Source: CAD feature listing. Evaluate the final solid. Frame: model axes, mm. A direction names the side the tool comes from. Coordinates: 2 decimals unless noted, no trailing zeros. Write each loop counter-clockwise with the first axis right and the second up, starting at its lowest first coordinate (ties: lowest second). Pieces come first, ordered by that corner, then holes. Notation, with made-up numbers: (4.25, 61) -> (58.25, 61) arc R16 cw to (58.25, 86) -> close; hole circle Ø4 at (38.5, 62.5). An arc over 180 degrees is marked (long way). Write item = value, one per line.
from build123d import *

# Parameters (mm, degrees)
SKETCH1_W           = 125
SKETCH1_H           = 125
SKETCH1_W_2         = 121
SKETCH1_H_2         = 121
BOSS_EXTRUDE1_DEPTH = 70
SKETCH2_W           = 125
SKETCH2_H           = 125
BOSS_EXTRUDE2_DEPTH = 2
SKETCH3_R           = 1.5
CUT_EXTRUDE1_DEPTH  = 3
FILLET2_R           = 3
FILLET3_R           = 3
CUT_EXTRUDE2_REACH  = 158.305
SKETCH4_R           = 11.1
SKETCH4_R_2         = 10
CUT_EXTRUDE3_REACH  = 158.305
SKETCH5_R           = 1.5


with BuildPart() as part:
    # Sketch1 → Boss-Extrude1 (new body)
    with BuildSketch(Plane(origin=(0, 0, 0), x_dir=(1, 0, 0), z_dir=(0, 1, 0))):
        Rectangle(SKETCH1_W, SKETCH1_H)
        Rectangle(SKETCH1_W_2, SKETCH1_H_2, mode=Mode.SUBTRACT)
    extrude(amount=BOSS_EXTRUDE1_DEPTH)

    # Sketch2 → Boss-Extrude2 (add)
    with BuildSketch(Plane.XZ):
        Rectangle(SKETCH2_W, SKETCH2_H)
    extrude(amount=BOSS_EXTRUDE2_DEPTH)

    # Sketch3 → Cut-Extrude1 (cut)
    with BuildSketch(Plane.XZ.offset(2)):
        with Locations(Location((38, -32.5, 0), (0, 0, 270))):
            Circle(SKETCH3_R)
        with Locations(Location((-38, -32.5, 0), (0, 0, 270))):
            Circle(SKETCH3_R)
        with Locations(Location((38, 32.5, 0), (0, 0, 270))):
            Circle(SKETCH3_R)
        with Locations(Location((-38, 32.5, 0), (0, 0, 270))):
            Circle(SKETCH3_R)
    extrude(amount=-CUT_EXTRUDE1_DEPTH, mode=Mode.SUBTRACT)

    # Fillet2
    fillet2_edges = [part.edges().sort_by_distance(p)[0] for p in [
        (-62.5, -2, 0),
        (0, -2, -62.5),
        (62.5, -2, 0),
        (0, -2, 62.5),
    ]]
    fillet(fillet2_edges, radius=FILLET2_R)

    # Fillet3
    fillet3_edges = [part.edges().sort_by_distance(p)[0] for p in [
        (-60.5, 0, 0),
        (0, 0, 60.5),
        (60.5, 0, 0),
        (0, 0, -60.5),
    ]]
    fillet(fillet3_edges, radius=FILLET3_R)

    # Sketch4 → Cut-Extrude2 (cut, up to next)
    with BuildSketch(Plane.XY.offset(62.5), mode=Mode.PRIVATE) as cut_extrude2_sk1:
        with Locations((0, 17)):
            Circle(SKETCH4_R)
    cut_extrude2_tool1 = extrude(cut_extrude2_sk1.sketch, amount=-CUT_EXTRUDE2_REACH, mode=Mode.PRIVATE) & part.part
    # Sketch4 → Cut-Extrude2 (cut, up to next)
    with BuildSketch(Plane.XY.offset(62.5), mode=Mode.PRIVATE) as cut_extrude2_sk2:
        with Locations((0, 43)):
            Circle(SKETCH4_R_2)
    cut_extrude2_tool2 = extrude(cut_extrude2_sk2.sketch, amount=-CUT_EXTRUDE2_REACH, mode=Mode.PRIVATE) & part.part
    add(cut_extrude2_tool1.solids().sort_by_distance((0, 17, 62.5))[0], mode=Mode.SUBTRACT)
    add(cut_extrude2_tool2.solids().sort_by_distance((0, 43, 62.5))[0], mode=Mode.SUBTRACT)

    # Sketch5 → Cut-Extrude3 (cut, up to next)
    with BuildSketch(Plane.XY.offset(62.5), mode=Mode.PRIVATE) as cut_extrude3_sk1:
        with Locations((-15, 43)):
            Circle(SKETCH5_R)
    cut_extrude3_tool1 = extrude(cut_extrude3_sk1.sketch, amount=-CUT_EXTRUDE3_REACH, mode=Mode.PRIVATE) & part.part
    # Sketch5 → Cut-Extrude3 (cut, up to next)
    with BuildSketch(Plane.XY.offset(62.5), mode=Mode.PRIVATE) as cut_extrude3_sk2:
        with Locations(Location((15, 43, 0), (0, 0, 180))):
            Circle(SKETCH5_R)
    cut_extrude3_tool2 = extrude(cut_extrude3_sk2.sketch, amount=-CUT_EXTRUDE3_REACH, mode=Mode.PRIVATE) & part.part
    add(cut_extrude3_tool1.solids().sort_by_distance((-15, 43, 62.5))[0], mode=Mode.SUBTRACT)
    add(cut_extrude3_tool2.solids().sort_by_distance((15, 43, 62.5))[0], mode=Mode.SUBTRACT)


solid = part.part
1) Cut plane B-B, the plane z = 55. Output: boundary loops of the cut face in (x, y), and give its area (3 significant figures).
Answer block:
outline = (-62.5, 1) arc R3 ccw to (-59.5, -2) -> (59.5, -2) arc R3 ccw to (62.5, 1) -> (62.5, 70) -> (60.5, 70) -> (60.5, 3) arc R3 cw to (57.5, 0) -> (-57.5, 0) arc R3 cw to (-60.5, 3) -> (-60.5, 70) -> (-62.5, 70) -> close
area = 530 mm2
2) Reachability of faces 1 (the flat face through (-1, 29, 60.5)), 2 (the cylindrical face through (0.88, -1.14, 61.6)), 3 (the cylindrical face through (-15.325, 41.536, 61.514)) from +Z, -Z, +X, -X, +Y, -Y: full face, straight path, thin tool, end or side. Return the list, or none.
Answer block:
face_1 = +Y
face_2 = +Z, +X, -X, -Y
face_3 = +Z
3) Cut plane A-A, the plane x = 3. Output: boundary loops of the cut face in (y, z).
Answer block:
outline = (-2, -59.5) arc R3 ccw to (1, -62.5) -> (70, -62.5) -> (70, -60.5) -> (3, -60.5) arc R3 cw to (0, -57.5) -> (0, 57.5) arc R3 cw to (3, 60.5) -> (6.31, 60.5) -> (6.31, 62.5) -> (1, 62.5) arc R3 ccw to (-2, 59.5) -> close; (27.69, 60.5) -> (33.46, 60.5) -> (33.46, 62.5) -> (27.69, 62.5) -> close; (52.54, 60.5) -> (70, 60.5) -> (70, 62.5) -> (52.54, 62.5) -> close
4) Material intervals for probe 1 along Y at (x, z) = (0, 62); probe 2 along Z at (x, y) = (-41, 50.5), sorted ascending. Write a range as [from, to].
Answer block:
probe_1 = [-0.66, 5.9], [28.1, 33], [53, 70]
probe_2 = [-62.5, -60.5], [60.5, 62.5]
5) Cut plane C-C, the plane x = 19. Output: boundary loops of the cut face in (y, z).
Answer block:
outline = (-2, -59.5) arc R3 ccw to (1, -62.5) -> (70, -62.5) -> (70, -60.5) -> (3, -60.5) arc R3 cw to (0, -57.5) -> (0, 57.5) arc R3 cw to (3, 60.5) -> (70, 60.5) -> (70, 62.5) -> (1, 62.5) arc R3 ccw to (-2, 59.5) -> close
6) Pull-direction query (Y, two-part tool) for faces 4 (the flat face through (-0.9, 28.3, 62.5)), 5 (the cylindrical face through (-8.81, 10.25, 61.51)), 6 (the cylindrical face through (0.88, -1.14, -61.6)), 7 (the cylindrical face through (-2.17, 33.24, 61.51)); classes: +Y half, -Y half, draft (parallel to the pull), parting line (faces both ways), or undercut.
Answer block:
face_4 = draft
face_5 = undercut
face_6 = -Y half
face_7 = undercut
7) First-contact query: pin 1 Ø3.5 at (x, y) = (-15, 43) entering from +Z; pin 2 Ø6 at (x, z) = (32, -11.5) entering from +Y; pin 3 Ø1.8 at (x, z) = (-38, -32.5) entering from -Y; pin 4 Ø18 at (x, y) = (0, 43) entering from +Z. Flat tips, straight axial feed; report the tip coordinate or a pass-through.
Answer block:
pin_1 = 62.5
pin_2 = 0
pin_3 = through
pin_4 = -60.5
